Geometry: final body of the model. Coordinates: model frame, mm. A direction names the side the tool comes from. Give positions to 0.01 mm unless a question says otherwise; leave off trailing zeros. Order: outer loops, then holes, each group sorted by start corner. A loop starts at its lowest first (then second) coordinate and runs counter-clockwise, first axis right, second up. Notation, with made-up numbers: (46, 74) -> (99, 74) arc R30 cw to (99, 102) -> close; hole circle Ø4 at (20.25, -7). An arc over 180 degrees is marked (long way). One line per question, with ' | ' between items. Start each with the question number.
(1) Mould query, pull axis Z, two halves, no side actions, for faces 1 (the face through (13, 5, -10.5)), 2 (the face through (31, 5, 0)), 3 (the face through (38.968, 7.042, -1.425)). Classes: +Z half, -Z half, draft (parallel to the pull), parting line (faces both ways), or undercut.
(2) First-contact query: pin 1 Ø8 at (x, y) = (-25, 4) entering from +Z; pin 2 Ø2.5 at (x, z) = (-27, -29) entering from +Y; pin 3 Ø6.5 at (x, z) = (37.5, -1) entering from +Y. Flat tips, straight axial feed; report the tip coordinate or a pass-through.
(3) Section A-A (y = 6.25). State how many separate pieces and enclosed holes the cut face has, then the cut area to 3 significant figures.
(4) Ray query, L1, parallel to Z at x = 36.5, y = 1.35; L2, parallel to X at y = 3.1, z = 0; L3, parallel to Y at x = -27, z = -24.5. Return the intervals inside material, ascending.
(5) Set-up query: faces 4 (the face through (-44.796, 6.072, -10.356)), 5 (the face through (38, 4, -1)), 6 (the face through (0, 5, -5.5)). Return all of +Z, -Z, +X, -X, +Y, -Y with unobstructed straight access to the full face (end or side cutting, diameter ignored); none if empty.
(6) Section D-D (x = 17.5). Return loops of the section in (y, z), then the cut area to 3 significant figures.
(7) Section B-B (x = 36.5). Return loops of the section in (y, z), then the cut area to 3 significant figures.
```python
from build123d import *

# Parameters (mm, degrees)
EXTRUDE_1_DEPTH          = 10
SKETCH_2_R               = 1.5
CUT_EXTRUDE_1_DEPTH      = 10
CUT_EXTRUDE_2_DEPTH      = 6
EXTRUDE_2_DEPTH          = 16
CUT_EXTRUDE_3_DEPTH      = 60.059147092
CUT_EXTRUDE_3_DEPTH_BACK = 36.4308247
SKETCH_6_R               = 3.5
CUT_EXTRUDE_4_DEPTH      = 36.4308247
SKETCH_8_R               = 5.25
CUT_EXTRUDE_6_DEPTH      = 24


with BuildPart() as part:
    # 草图1 → 凸台-拉伸1 (new body)
    with BuildSketch(Plane(origin=(0, 0, 0), x_dir=(1, 0, 0), z_dir=(0, 1, 0))):
        Polygon((-42, 5.5), (-42, 10.5), (42, 10.5), (42, 5.5), (42, -5.5), (31, -5.5), (31, 5.5), (-31, 5.5), (-31, -5.5), (-42, -5.5), align=None)
    extrude(amount=EXTRUDE_1_DEPTH)

    # 草图2 → 切除-拉伸1 (cut)
    with BuildSketch(Plane(origin=(0, 10, 0), x_dir=(1, 0, 0), z_dir=(0, 1, 0))):
        with Locations((-36.5, 0)):
            Circle(SKETCH_2_R)
        with Locations((36.5, 0)):
            Circle(SKETCH_2_R)
    extrude(amount=-CUT_EXTRUDE_1_DEPTH, mode=Mode.SUBTRACT)

    # 草图3 → 切除-拉伸2 (cut)
    with BuildSketch(Plane(origin=(0, 10, 0), x_dir=(1, 0, 0), z_dir=(0, 1, 0))):
        Polygon((-34.826211876, -2.833449014), (-33.209267111, 0.032818529), (-34.883055236, 2.866267543), (-38.173788124, 2.833449014), (-39.790732889, -0.032818529), (-38.116944764, -2.866267543), align=None)
        Polygon((38.168661206, -2.836471361), (39.790786858, 0.026867314), (38.122125653, 2.863338675), (34.831338794, 2.836471361), (33.209213142, -0.026867314), (34.877874347, -2.863338675), align=None)
    extrude(amount=-CUT_EXTRUDE_2_DEPTH, mode=Mode.SUBTRACT)

    # 草图4 → 凸台-拉伸2 (add)
    with BuildSketch(Plane(origin=(0, 0, 0), x_dir=(1, 0, 0), z_dir=(0, 1, 0))):
        Polygon((-44.778370843, 26.256924048), (-47.514531989, 25.774465014), (-42, -5.5), (-42, 10.5), (-14.358361399, 10.5), (-17.970229632, 30.983922646), align=None)
    extrude(amount=EXTRUDE_2_DEPTH)

    # 草图5 → 切除-拉伸3 (cut, two sides)
    with BuildSketch(Plane(origin=(-12.129798074, 0, 2.138810671), x_dir=(-0.173648178, 0, -0.984807753), z_dir=(0.984807753, 0, -0.173648178))) as cut_extrude_3_sk:
        with BuildLine():
            Line((33.533704869, 8), (33.633704869, 8))
            Line((33.633704869, 8), (33.633704869, 16))
            Line((33.633704869, 16), (1.87678082, 16))
            Line((1.87678082, 16), (1.87678082, 10))
            Line((1.87678082, 10), (12.833784698, 10))
            Line((12.833784698, 10), (17.991061347, 10))
            ThreePointArc((17.991061347, 10), (26.641949923, 15.83539673), (33.533704869, 8))
        make_face()
    extrude(amount=CUT_EXTRUDE_3_DEPTH, mode=Mode.SUBTRACT)
    extrude(cut_extrude_3_sk.sketch, amount=-CUT_EXTRUDE_3_DEPTH_BACK, mode=Mode.SUBTRACT)

    # 草图6 → 切除-拉伸4 (cut, through all)
    with BuildSketch(Plane(origin=(-12.129798074, 0, 2.138810671), x_dir=(-0.173648178, 0, -0.984807753), z_dir=(0.984807753, 0, -0.173648178))):
        with Locations((25.633704869, 8)):
            Circle(SKETCH_6_R)
    extrude(amount=-CUT_EXTRUDE_4_DEPTH, mode=Mode.SUBTRACT)

    # 草图8 → 切除-拉伸6 (cut)
    with BuildSketch(Plane(origin=(-41.674100431, 0, 7.348268303), x_dir=(0.173648178, 0, 0.984807753), z_dir=(-0.984807753, 0, 0.173648178))):
        with Locations((-25.633704869, 8)):
            Circle(SKETCH_8_R)
    extrude(amount=-CUT_EXTRUDE_6_DEPTH, mode=Mode.SUBTRACT)


solid = part.part
```
Response:
1) face 1: -Z half | face 2: draft | face 3: undercut
2) pin 1: stops at z = -5.5 | pin 2: stops at y = 12.68 | pin 3: stops at y = 10
3) separate pieces: 2 | enclosed holes: 2 | area: 899 mm^2
4) L1: z = -10.5 to -1.5, 1.5 to 5.5 | L2: x = -42.97 to -38, -35 to -31, 31 to 35, 38 to 42 | L3: y = 0 to 3.82, 12.18 to 15.23
5) face 4: +Z, -X, +Y, -Y | face 5: +Y | face 6: +Z, +Y, -Y
6) outline: (0, -10.5) -> (10, -10.5) -> (10, -5.5) -> (0, -5.5) -> close | area: 50.0 mm^2
7) outline: (0, -10.5) -> (10, -10.5) -> (10, -2.85) -> (4, -2.85) -> (4, -1.5) -> (0, -1.5) -> close; (0, 1.5) -> (4, 1.5) -> (4, 2.85) -> (10, 2.85) -> (10, 5.5) -> (0, 5.5) -> close | area: 114 mm^2
